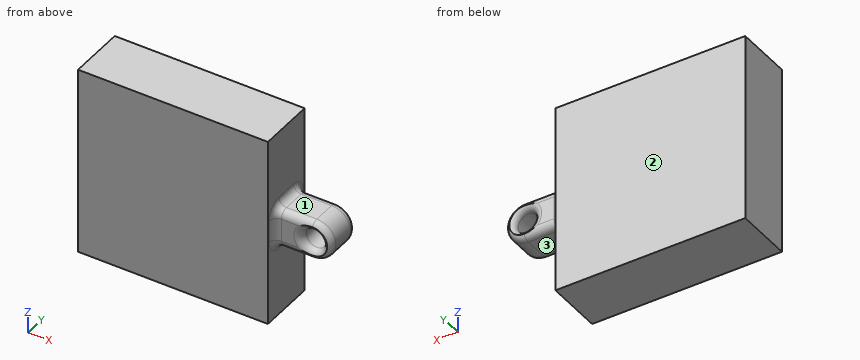
Autodesk Inventor part; units mm, degrees
ref_plane "YZ Plane" through (0, 0, 0) normal (1, 0, 0) x (0, 1, 0)
ref_plane "XZ Plane" through (0, 0, 0) normal (0, 1, 0) x (-1, 0, 0)
ref_plane "XY Plane" through (0, 0, 0) normal (0, 0, 1) x (1, 0, 0)
sketch "Sketch1" plane through (0, 0, 0) normal (0, 1, 0) x (-1, 0, 0)
  line L0 (0, 0) -> (-50, 0)
  line L1 (-50, 0) -> (-50, -50)
  line L2 (-50, -50) -> (0, -50)
  line L3 (0, -50) -> (0, 0)
  dimension "d0" = 50
  dimension "d1" = 50
extrude "Extrusion1" add sketch "Sketch1" along normal blind 15
ref_plane "Work Plane1" through (0, 7.5, 0) normal (0, 1, 0) x (1, 0, 0)
sketch "Sketch2" plane through (0, 7.5, 0) normal (0, 1, 0) x (1, 0, 0)
  line L0 (50, 20) -> (60, 20)
  line L1 (60, 20) -> (60, 30) construction
  line L2 (60, 30) -> (50, 30)
  line L3 (50, 30) -> (50, 20)
  line L4 (50, 20) -> (60, 30) construction
  line L5 (60, 20) -> (50, 30) construction
  line L6 (50, 0) -> (50, 50)
  arc A0 (60, 20) -> (60, 30) centre (60, 25) ccw
  line L7 (50, 25) -> (60, 25) construction
  point P0 (0, 0)
  dimension "d4" = 10
  dimension "d5" = 10
extrude "Extrusion2" add sketch "Sketch2" along normal mid plane 10
sketch "Sketch3" plane through (0, 12.5, 0) normal (0, 1, 0) x (1, 0, 0)
  arc A0 (60, 20) -> (60, 30) centre (60, 25) ccw
  point P0 (0, 0)
hole "Hole1" at (60, 12.5, -25) direction (0, -1, 0) diameter 5.5 end through all
fillet "Fillet1" radius 2 12 edges at (55, 2.5, -20) (55, 2.5, -30) (65, 2.5, -25) (55, 12.5, -30) (55, 12.5, -20) (65, 12.5, -25) (60, 12.5, -27.75) (60, 2.5, -27.75) (50, 12.5, -25) (50, 7.5, -20) (50, 2.5, -25) (50, 7.5, -30)
properties part number "Casing_Part3"
Model file for the job. Use its own axes, mm. Face numbers are marked on the shaded views. A direction names the side the tool comes from. Give positions to 0.01 mm unless a question says otherwise; leave off trailing zeros. Order: outer loops, then holes, each group sorted by start corner. A loop starts at its lowest first (then second) coordinate and runs counter-clockwise, first axis right, second up. Notation, with made-up numbers: M 23,28.5 L 50,28.5 A6 cw 50,35.5 Z; hole C 79.5,36 d4. An arc over 180 degrees is marked long. Put each result on its own line as item: value. Start each with the question number.
(1) Band-saw the part on A-A on z = -25. Give the cut face in (x, y) (3 decimals).
(2) Band-saw the part on B-B on z = -46. Give the cut face in (x, y).
(3) Tool access for the marked faces 1, 2 and 3: list every direction of +Z, -Z, +X, -X, +Y, -Y with a clear straight run to the whole face (end or side of a thin tool).
(4) Pin check, flat tips, straight feed: pin 1 Ø6.5 at (x, y) = (56.5, 9) entering from -Z; pin 2 Ø2 at (x, z) = (54, -24.5) entering from +Y; pin 3 Ø2 at (y, z) = (9, -28) entering from +X. Stop position of each tip, or through.
(5) Drill centre lines: L1, parallel to Z at x = 60, y = 7.75; L2, parallel to X at y = 6.2, z = -25; L3, parallel to X at y = 12.25, z = -22.5. Where is each one in solid material? Low to high. Write a range as [from, to].
Results below:
1. outline: M 0,0 L 50,0 L 50,0.5 A2 cw 52,2.5 L 55.25,2.5 A2 ccw 57.25,4.5 L 57.25,10.5 A2 ccw 55.25,12.5 L 52,12.5 A2 cw 50,14.5 L 50,15 L 0,15 Z; M 62.75,4.5 A2 ccw 63.875,2.702 A2 ccw 65,4.5 L 65,10.5 A2 ccw 63.875,12.298 A2 ccw 62.75,10.5 Z
2. outline: M 0,0 L 50,0 L 50,15 L 0,15 Z
3. face 1: +Z, +X, +Y, -Y
3. face 2: +Z, -Z, +X, -X, +Y
3. face 3: -Z, +X, +Y, -Y
4. pin 1: stops at z = -30
4. pin 2: stops at y = 12.5
4. pin 3: stops at x = 64.58
5. L1: z = [-30, -27.75], [-22.25, -20]
5. L2: x = [0, 57.25], [62.75, 65]
5. L3: x = [0, 57.16], [62.84, 63.08]
